```python
from build123d import *

# Parameters (mm, degrees)
BOSS_EXTRUDE1_DEPTH = 15.24
SKETCH2_R           = 2.38125
CUT_EXTRUDE1_DEPTH  = 15.24
CHAMFER1_SIZE       = 8.89
SKETCH3_R           = 3.175
CUT_EXTRUDE2_DEPTH  = 7.9375
SKETCH4_R           = 3.175
CUT_EXTRUDE3_DEPTH  = 7.9375


with BuildPart() as part:
    # Sketch1 → Boss-Extrude1 (new body)
    with BuildSketch(Plane(origin=(0, 0, 0), x_dir=(1, 0, 0), z_dir=(0, 1, 0))):
        Polygon((-241.141854356, 15.046517442), (-241.141854356, 94.421517442), (-203.041854356, 108.709017442), (-50.641854356, 108.709017442), (114.335985065, 203.959017442), (368.335985065, 203.959017442), (622.335985065, 203.959017442), (787.313824486, 108.709017442), (939.713824486, 108.709017442), (977.813824486, 94.421517442), (977.813824486, 15.046517442), (939.713824486, 0.759017442), (787.313824486, 0.759017442), (622.335985065, -94.490982558), (368.335985065, -94.490982558), (114.335985065, -94.490982558), (-50.641854356, 0.759017442), (-203.041854356, 0.759017442), align=None)
    extrude(amount=BOSS_EXTRUDE1_DEPTH)

    # Sketch2 → Cut-Extrude1 (cut)
    with BuildSketch(Plane(origin=(0, 0, 0), x_dir=(-1, 0, 0), z_dir=(0, -1, 0))):
        with Locations(Location((182.721854356, 34.096517442, 0), (0, 0, 90))):
            Circle(SKETCH2_R)
        with Locations(Location((182.721854356, 75.371517443, 0), (0, 0, 90))):
            Circle(SKETCH2_R)
        with Locations(Location((119.221854356, 75.371517443, 0), (0, 0, 90))):
            Circle(SKETCH2_R)
        with Locations(Location((119.221854356, 34.096517443, 0), (0, 0, 90))):
            Circle(SKETCH2_R)
        with Locations(Location((-855.893824486, 75.371517443, 0), (0, 0, 90))):
            Circle(SKETCH2_R)
        with Locations(Location((-919.393824486, 75.371517443, 0), (0, 0, 90))):
            Circle(SKETCH2_R)
        with Locations(Location((-919.393824486, 34.096517442, 0), (0, 0, 90))):
            Circle(SKETCH2_R)
        with Locations(Location((-855.893824486, 34.096517443, 0), (0, 0, 90))):
            Circle(SKETCH2_R)
    extrude(amount=-CUT_EXTRUDE1_DEPTH, mode=Mode.SUBTRACT)

    # Chamfer1
    chamfer1_edges = [part.edges().sort_by_distance(p)[0] for p in [
        (-126.841854356, 0, -0.759017442),
        (-222.091854356, 0, -7.902767442),
        (-241.141854356, 0, -54.734017442),
        (-222.091854356, 0, -101.565267442),
        (-126.841854356, 0, -108.709017442),
        (31.847065354, 0, -156.334017442),
        (368.335985065, 0, -203.959017442),
        (704.824904775, 0, -156.334017442),
        (863.513824486, 0, -108.709017442),
        (958.763824486, 0, -101.565267442),
        (977.813824486, 0, -54.734017442),
        (958.763824486, 0, -7.902767442),
        (863.513824486, 0, -0.759017442),
        (704.824904775, 0, 46.865982558),
        (368.335985065, 0, 94.490982558),
        (31.847065354, 0, 46.865982558),
    ]]
    chamfer(chamfer1_edges, length=CHAMFER1_SIZE)

    # Sketch3 → Cut-Extrude2 (cut)
    with BuildSketch(Plane.XZ):
        with Locations(Location((955.588824486, -80.134017442, 0), (0, 0, 270))):
            Circle(SKETCH3_R)
        with Locations(Location((955.588824486, -29.334017442, 0), (0, 0, 270))):
            Circle(SKETCH3_R)
        with Locations(Location((546.135985065, -156.334017442, 0), (0, 0, 270))):
            Circle(SKETCH3_R)
        with Locations(Location((482.635985065, -156.334017442, 0), (0, 0, 270))):
            Circle(SKETCH3_R)
        with Locations(Location((546.135985065, -105.534017442, 0), (0, 0, 270))):
            Circle(SKETCH3_R)
        with Locations(Location((482.635985065, -105.534017442, 0), (0, 0, 270))):
            Circle(SKETCH3_R)
        with Locations(Location((546.135985065, -80.134017442, 0), (0, 0, 270))):
            Circle(SKETCH3_R)
        with Locations(Location((546.135985065, -29.334017442, 0), (0, 0, 270))):
            Circle(SKETCH3_R)
        with Locations(Location((482.635985065, -29.334017442, 0), (0, 0, 270))):
            Circle(SKETCH3_R)
        with Locations(Location((482.635985065, -80.134017442, 0), (0, 0, 270))):
            Circle(SKETCH3_R)
        with Locations(Location((546.135985065, -3.934017442, 0), (0, 0, 270))):
            Circle(SKETCH3_R)
        with Locations(Location((546.135985065, 46.865982558, 0), (0, 0, 270))):
            Circle(SKETCH3_R)
        with Locations(Location((482.635985065, 46.865982558, 0), (0, 0, 270))):
            Circle(SKETCH3_R)
        with Locations(Location((482.635985065, -3.934017442, 0), (0, 0, 270))):
            Circle(SKETCH3_R)
        with Locations(Location((730.285985065, -54.734017442, 0), (0, 0, 270))):
            Circle(SKETCH3_R)
        with Locations(Location((730.285985065, -105.534017442, 0), (0, 0, 270))):
            Circle(SKETCH3_R)
        with Locations(Location((730.285985065, -3.934017442, 0), (0, 0, 270))):
            Circle(SKETCH3_R)
        with Locations(Location((711.235985065, 8.765982558, 0), (0, 0, 270))):
            Circle(SKETCH3_R)
        with Locations(Location((660.435985065, 8.765982558, 0), (0, 0, 270))):
            Circle(SKETCH3_R)
        with Locations(Location((622.335985065, -156.334017442, 0), (0, 0, 270))):
            Circle(SKETCH3_R)
        with Locations(Location((404.848485065, -156.334017442, 0), (0, 0, 270))):
            Circle(SKETCH3_R)
        with Locations(Location((404.848485065, -105.534017442, 0), (0, 0, 270))):
            Circle(SKETCH3_R)
        with Locations(Location((404.848485065, -54.734017442, 0), (0, 0, 270))):
            Circle(SKETCH3_R)
        with Locations(Location((404.848485065, -3.934017442, 0), (0, 0, 270))):
            Circle(SKETCH3_R)
        with Locations(Location((404.848485065, 46.865982558, 0), (0, 0, 270))):
            Circle(SKETCH3_R)
        with Locations(Location((660.435985065, -118.234017442, 0), (0, 0, 90))):
            Circle(SKETCH3_R)
        with Locations(Location((711.235985065, -118.234017442, 0), (0, 0, 90))):
            Circle(SKETCH3_R)
        with Locations(Location((641.385985065, -105.534017442, 0), (0, 0, 90))):
            Circle(SKETCH3_R)
        with Locations(Location((641.385985065, -54.734017442, 0), (0, 0, 90))):
            Circle(SKETCH3_R)
        with Locations(Location((641.385985065, -3.934017442, 0), (0, 0, 270))):
            Circle(SKETCH3_R)
        with Locations(Location((622.335985065, -105.534017442, 0), (0, 0, 270))):
            Circle(SKETCH3_R)
        with Locations(Location((622.335985065, -54.734017442, 0), (0, 0, 270))):
            Circle(SKETCH3_R)
        with Locations(Location((622.335985065, -3.934017442, 0), (0, 0, 270))):
            Circle(SKETCH3_R)
        with Locations(Location((622.335985065, 46.865982558, 0), (0, 0, 270))):
            Circle(SKETCH3_R)
        with Locations(Location((601.698485065, -181.734017442, 0), (0, 0, 270))):
            Circle(SKETCH3_R)
        with Locations(Location((550.898485065, -181.734017442, 0), (0, 0, 270))):
            Circle(SKETCH3_R)
        with Locations(Location((500.098485065, -181.734017443, 0), (0, 0, 270))):
            Circle(SKETCH3_R)
        with Locations(Location((449.298485065, -181.734017443, 0), (0, 0, 270))):
            Circle(SKETCH3_R)
        with Locations(Location((398.498485065, -181.734017443, 0), (0, 0, 270))):
            Circle(SKETCH3_R)
        with Locations(Location((398.498485065, 72.265982558, 0), (0, 0, 90))):
            Circle(SKETCH3_R)
        with Locations(Location((449.298485065, 72.265982558, 0), (0, 0, 90))):
            Circle(SKETCH3_R)
        with Locations(Location((500.098485065, 72.265982558, 0), (0, 0, 90))):
            Circle(SKETCH3_R)
        with Locations(Location((550.898485065, 72.265982558, 0), (0, 0, 90))):
            Circle(SKETCH3_R)
        with Locations(Location((601.698485065, 72.265982558, 0), (0, 0, 90))):
            Circle(SKETCH3_R)
        with Locations(Location((377.860985065, -156.334017442, 0), (0, 0, 90))):
            Circle(SKETCH3_R)
        with Locations(Location((377.860985065, -105.534017442, 0), (0, 0, 90))):
            Circle(SKETCH3_R)
        with Locations(Location((377.860985065, -54.734017442, 0), (0, 0, 90))):
            Circle(SKETCH3_R)
        with Locations(Location((377.860985065, -3.934017442, 0), (0, 0, 90))):
            Circle(SKETCH3_R)
        with Locations(Location((377.860985065, 46.865982558, 0), (0, 0, 90))):
            Circle(SKETCH3_R)
        with Locations(Location((936.538824486, -29.334017442, 0), (0, 0, 270))):
            Circle(SKETCH3_R)
        with Locations(Location((936.538824486, -80.134017442, 0), (0, 0, 270))):
            Circle(SKETCH3_R)
    extrude(amount=-CUT_EXTRUDE2_DEPTH, mode=Mode.SUBTRACT)

    # Sketch4 → Cut-Extrude3 (cut)
    with BuildSketch(Plane(origin=(0, 15.24, 0), x_dir=(1, 0, 0), z_dir=(0, 1, 0))):
        with Locations(Location((939.713824486, 89.761899088, 0), (0, 0, 270.000000003))):
            Circle(SKETCH4_R)
        with Locations(Location((939.713824486, 19.706135797, 0), (0, 0, 90))):
            Circle(SKETCH4_R)
        with Locations(Location((888.913824486, 89.761899088, 0), (0, 0, 270.000000002))):
            Circle(SKETCH4_R)
        with Locations(Location((888.913824486, 19.706135797, 0), (0, 0, 90))):
            Circle(SKETCH4_R)
        with Locations(Location((838.113824486, 89.761899088, 0), (0, 0, 270.000000002))):
            Circle(SKETCH4_R)
        with Locations(Location((838.113824486, 19.706135797, 0), (0, 0, 90))):
            Circle(SKETCH4_R)
        with Locations(Location((787.313824486, 89.761899088, 0), (0, 0, 270.000000002))):
            Circle(SKETCH4_R)
        with Locations(Location((787.313824486, 19.706135797, 0), (0, 0, 90))):
            Circle(SKETCH4_R)
        with Locations(Location((774.613824486, 54.734017442, 0), (0, 0, 270))):
            Circle(SKETCH4_R)
        with Locations(Location((952.413824486, 45.209017442, 0), (0, 0, 90))):
            Circle(SKETCH4_R)
        with Locations(Location((952.413824486, 64.259017442, 0), (0, 0, 270))):
            Circle(SKETCH4_R)
    extrude(amount=-CUT_EXTRUDE3_DEPTH, mode=Mode.SUBTRACT)


solid = part.part
```
Design review of the part built by this model. Coordinates are the model's own, in mm. Coordinates: 2 decimals unless noted, no trailing zeros. Loops run counter-clockwise (first coordinate to the right, second up) from the corner with the lowest first, then second, coordinate; pieces in that order, holes last. Notation, with made-up numbers: (82, 63) -> (132, 63) arc R13 ccw to (132, 78) -> close; hole circle Ø8 at (63.25, 24). An arc over 180 degrees is marked (long way). Answer as a JSON object with one key per item and string values.
Q1. Clearance check with flat-ended pins moving along their axes: pin 1 Ø10 at (x, z) = (955.59, -29.33) entering from -Y; pin 2 Ø5 at (x, y) = (-159, 10.5) entering from -Z; pin 3 Ø4 at (x, y) = (670.5, 12) entering from +Z; pin 4 Ø1 at (y, z) = (2, -50) entering from +X. State where each tip first meets the part, or that it passes through.
Answer block:
{"pin 1": "stops at y = 0", "pin 2": "stops at z = -108.71", "pin 3": "stops at z = 67.84", "pin 4": "stops at x = 971.42"}
Q2. The part is to be moulded in two halves that separate along X. For faces 1 (the flat face through (702.5, 4.51, -152.62)), 2 (the flat face through (377, 0, -26)), 3 (the flat face through (34.176, 4.507, 43.15)), say which applies: +X half, -X half, draft (parallel to the pull), parting line (faces both ways), or undercut.
Answer block:
{"face 1": "+X half", "face 2": "draft", "face 3": "-X half"}
Q3. Take a section at A-A on x = 338. Give the boundary of the cut face in (y, z).
Answer block:
{"outline": "(0, -195.07) -> (8.89, -203.96) -> (15.24, -203.96) -> (15.24, 94.49) -> (8.89, 94.49) -> (0, 85.6) -> close"}
Q4. Take a section at B-B on y = 3.75. Give the number of separate pieces and of enclosed holes in the cut face, plus the area to 3 significant figures.
Answer block:
{"separate pieces": "1", "enclosed holes": "59", "area": "243,000 mm^2"}
Q5. Take a section at C-C on z = 28.5. Give the boundary of the cut face in (x, y).
Answer block:
{"outline": "(0.04, 8.89) -> (17.82, 0) -> (718.86, 0) -> (736.64, 8.89) -> (736.64, 15.24) -> (0.04, 15.24) -> close"}
Q6. To check wall thickness, follow L1, parallel to X at y = 4.75, z = 49.5; L2, parallel to X at y = 1.75, z = -7.5; L3, parallel to Z at x = -38.5, y = 8.25. State the ranges of each line that lie inside material, in increasing order.
Answer block:
{"L1": "x = 44.69 to 376.09, 379.63 to 403.08, 406.62 to 480.86, 484.41 to 544.36, 547.91 to 620.56, 624.11 to 691.98", "L2": "x = -48.04 to 784.71", "L3": "z = -114.98 to 5.51"}
